```python
from build123d import *

# Parameters (mm, degrees)
F0_R     = 55
F1_DEPTH = 2
F2_R     = 1.5
F3_DEPTH = 25
F4_R     = 5
F5_DEPTH = 3


# Not quite as in the source:
# - a fillet or chamfer that OpenCascade refuses, or shapes differently, is made with other operations: its cross-section is extruded or revolved along the edge and cut away or added
# - a feature names something its author has since deleted; it is built from what else it names


with BuildPart() as f1:
    # F0 (on Top) → F1 (new body)
    with BuildSketch(Plane.XY):
        Circle(F0_R)
    extrude(amount=F1_DEPTH)

    # F2 (on face) → F3 (cut)
    with BuildSketch(Plane(origin=(0, 0, 0), x_dir=(1, 0, 0), z_dir=(0, 0, -1))):
        with Locations((-45, 0)):
            Circle(F2_R)
        with Locations((0, 45)):
            Circle(F2_R)
        with Locations((45, 0)):
            Circle(F2_R)
        with Locations((0, -45)):
            Circle(F2_R)
    extrude(amount=-F3_DEPTH, mode=Mode.SUBTRACT)

    # F4 (on face) → F5 (join)
    with BuildSketch(Plane.XY.offset(2)):
        with Locations((27, 0)):
            Circle(F4_R)
    extrude(amount=F5_DEPTH)

    # F6: chamfer of 5 on 1 edges, made by hand


with BuildPart() as f6_tool2:
    # F6_s3 → F6_t4 (revolve)
    with BuildSketch(Plane.XZ):
        Polygon((32, 0), (27, 5), (32, 5), align=None)
    revolve(axis=Axis((27, 0, 5), (0, 0, 1)))

    split(bisect_by=Plane.XY.offset(2), keep=Keep.TOP)


with BuildPart() as f1_1:
    add(f1.part)

    # F6_t1: cut F6_tool2
    add(f6_tool2.part, mode=Mode.SUBTRACT)


solid = f1_1.part
```
The model under review builds one solid part; all positions refer to its coordinate system, in mm. Round coordinates to 2 decimals unless told otherwise and drop trailing zeros. Order: outer loops, then holes, each group sorted by start corner. A loop starts at its lowest first (then second) coordinate and runs counter-clockwise, first axis right, second up. Notation, with made-up numbers: (65, -29.5) - (69, -29.5) arc R26 cw to (69, 5.5) - close; hole circle Ø8 at (9, 17). An arc over 180 degrees is marked (long way). Answer in a Markdown table with one row per item.
(1) Take a section at D-D on z = 3.3. Write out the cut boundary in (x, y).
Result set:
| item | result |
|---|---|
| outline | circle Ø3.4 at (27, 0) |
(2) Mouldability with a two-part tool opening along X and no side actions: class faces 1 (the face through (43.5, -0.07, 0.99)), 2 (the face through (-0.325, -43.536, 0.986)), 3 (the face through (-11.923, -53.692, 0.986)), 4 (the face through (-1, 1, 2)) as released by +X, released by -X, zero draft, split by the parting line, or undercut.
Result set:
| item | result |
|---|---|
| face 1 | undercut |
| face 2 | undercut |
| face 3 | split by the parting line |
| face 4 | zero draft |
(3) Take a section at B-B on y = -45. Write out the cut boundary in (x, z), plus the area to 3 significant figures.
Result set:
| item | result |
|---|---|
| outline | (-31.62, 0) - (-1.5, 0) - (-1.5, 2) - (-31.62, 2) - close; (1.5, 0) - (31.62, 0) - (31.62, 2) - (1.5, 2) - close |
| area | 120 mm2 |
(4) Clearance check with flat-ended pins moving along their axes: P1, Ø1.5, axis at x = 21.5, z = 2, coming from the +Y side; P2, Ø4, axis at x = 0, y = -45, coming from the +Z side; P3, Ø3, axis at x = -31.5, z = 2.5, coming from the -Y side. State where each tip first meets the part, or that it passes through.
Result set:
| item | result |
|---|---|
| P1 | stops at y = 50.94 |
| P2 | stops at z = 2 |
| P3 | stops at y = -46.04 |
(5) Take a section at A-A on x = 0. Write out the cut boundary in (y, z).
Result set:
| item | result |
|---|---|
| outline | (-55, 0) - (-46.5, 0) - (-46.5, 2) - (-55, 2) - close; (-43.5, 0) - (43.5, 0) - (43.5, 2) - (-43.5, 2) - close; (46.5, 0) - (55, 0) - (55, 2) - (46.5, 2) - close |
(6) For line 1 (Y direction, x = 0, z = 0.6); line 2 (Z direction, x = 3, y = 39.5); line 3 (Y direction, x = 45, z = 0.65), list the stretches that pass through material, from the lowest coordinate up. Write a range as from..to.
Result set:
| item | result |
|---|---|
| line 1 | y = -55..-46.5, -43.5..43.5, 46.5..55 |
| line 2 | z = 0..2 |
| line 3 | y = -31.62..-1.5, 1.5..31.62 |
